Here's how the part is built. I have some questions about the finished solid (model axes, mm). A direction names the side the tool comes from. Round coordinates to 2 decimals unless told otherwise and drop trailing zeros.
```python
from build123d import *

# Parameters (mm, degrees)
F0_W     = 100
F0_H     = 25
F1_DEPTH = 1
F2_W     = 0.8
F2_H     = 25
F2_W_2   = 0.9
F2_W_3   = 1
F2_W_4   = 1.1
F2_W_5   = 1.2
F2_W_6   = 1.3
F2_W_7   = 1.4
F2_W_8   = 1.5
F2_W_9   = 1.6
F2_W_10  = 1.7
F2_W_11  = 1.8
F2_W_12  = 1.9
F2_W_13  = 2
F2_W_14  = 2.1
F2_W_15  = 2.2
F2_W_16  = 2.3
F2_W_17  = 2.4
F2_W_18  = 2.5
F2_W_19  = 2.6
F2_W_20  = 2.7
F2_W_21  = 2.8
F2_W_22  = 2.9
F2_W_23  = 3
F3_DEPTH = 10
F4_W     = 23.160562
F4_H     = 27.70046
F5_DEPTH = 25


with BuildPart() as f1:
    # F0 (on Top) → F1 (new body)
    with BuildSketch(Plane.XY):
        with Locations((1.74681, -0.140128)):
            Rectangle(F0_W, F0_H)
    extrude(amount=F1_DEPTH)

    # F2 (on face) → F3 (join)
    with BuildSketch(Plane.XY.offset(1)):
        with Locations((-46.35319, -0.140128)):
            Rectangle(F2_W, F2_H)
        with Locations((-44.00319, -0.140128)):
            Rectangle(F2_W_2, F2_H)
        with Locations((-41.55319, -0.140128)):
            Rectangle(F2_W_3, F2_H)
        with Locations((-39.00319, -0.140128)):
            Rectangle(F2_W_4, F2_H)
        with Locations((-36.35319, -0.140128)):
            Rectangle(F2_W_5, F2_H)
        with Locations((-33.60319, -0.140128)):
            Rectangle(F2_W_6, F2_H)
        with Locations((-30.75319, -0.140128)):
            Rectangle(F2_W_7, F2_H)
        with Locations((-27.80319, -0.140128)):
            Rectangle(F2_W_8, F2_H)
        with Locations((-24.75319, -0.140128)):
            Rectangle(F2_W_9, F2_H)
        with Locations((-21.60319, -0.140128)):
            Rectangle(F2_W_10, F2_H)
        with Locations((-18.35319, -0.140128)):
            Rectangle(F2_W_11, F2_H)
        with Locations((-15.00319, -0.140128)):
            Rectangle(F2_W_12, F2_H)
        with Locations((-11.55319, -0.140128)):
            Rectangle(F2_W_13, F2_H)
        with Locations((-8.00319, -0.140128)):
            Rectangle(F2_W_14, F2_H)
        with Locations((-4.35319, -0.140128)):
            Rectangle(F2_W_15, F2_H)
        with Locations((-0.60319, -0.140128)):
            Rectangle(F2_W_16, F2_H)
        with Locations((3.24681, -0.140128)):
            Rectangle(F2_W_17, F2_H)
        with Locations((7.19681, -0.140128)):
            Rectangle(F2_W_18, F2_H)
        with Locations((11.24681, -0.140128)):
            Rectangle(F2_W_19, F2_H)
        with Locations((15.39681, -0.140128)):
            Rectangle(F2_W_20, F2_H)
        with Locations((19.64681, -0.140128)):
            Rectangle(F2_W_21, F2_H)
        with Locations((23.99681, -0.140128)):
            Rectangle(F2_W_22, F2_H)
        with Locations((28.44681, -0.140128)):
            Rectangle(F2_W_23, F2_H)
    extrude(amount=F3_DEPTH)

    # F4 (on face) → F5 (cut)
    with BuildSketch(Plane.XY.offset(1)):
        with Locations((43.004874, -0.135502)):
            Rectangle(F4_W, F4_H)
    extrude(amount=-F5_DEPTH, mode=Mode.SUBTRACT)


solid = f1.part
```
1) If we section it at A-A (z = 8): Give the number of separate pieces and of enclosed holes in the cut face, plus the area to 3 significant figures.
2) I need wall thicknesses on line 1 (Z direction, x = -35, y = -1). Which ranges of the line are inside material? Lowest first, please.
3) We'd pull the mould along X, two halves only. Please class faces 1 (the flat face through (-46.753, 0, 6)), 2 (the flat face through (-15.953, 0, 6)), 3 (the flat face through (-18, 12.36, 5)): +X half, -X half, draft (parallel to the pull), parting line (faces both ways), or undercut.
4) I'm going to push flat-ended pins straight in: pin 1 (5 mm diameter, centred on y = 4, z = 6.5, fed in from -X); pin 2 (3 mm diameter, centred on y = -3, z = 6.5, fed in from +X); pin 3 (0.8 mm diameter, centred on x = 5, y = -3, fed in from +Z). Where does each tip first touch, or does it pass through?
5) For faces 4 (the flat face through (2.047, 0, 6)), 5 (the flat face through (-12, 0, 11)), 6 (the flat face through (31, 0, 1)), which set-ups out of +Z, -Z, +X, -X, +Y, -Y let a thin tool reach every point of the face, with its end or its side?
Solutions:
1. separate pieces: 23
1. enclosed holes: 0
1. area: 1,090 mm2
2. line 1: z = 0 to 1
3. face 1: -X half
3. face 2: undercut
3. face 3: draft
4. pin 1: stops at x = -46.75
4. pin 2: stops at x = 29.95
4. pin 3: stops at z = 1
5. face 4: +Z, +Y, -Y
5. face 5: +Z, +X, -X, +Y, -Y
5. face 6: +Z, +X, +Y, -Y
